Build history of the part. All positions in model axes, mm. Face numbers are marked on the shaded views. Give positions to 0.01 mm unless a question says otherwise; leave off trailing zeros. Loops run counter-clockwise (first coordinate to the right, second up) from the corner with the lowest first, then second, coordinate; pieces in that order, holes last. Notation, with made-up numbers: M 72.25,17 L 98.25,17 A21 cw 98.25,41 Z; hole C 71.5,77.25 d9. An arc over 180 degrees is marked long. Put each result on its own line as item: value.
```python
from build123d import *

# Parameters (mm, degrees)
SKETCH1_R           = 2.5
BOSS_EXTRUDE1_DEPTH = 30
FILLET1_R           = 5


with BuildPart() as part:
    # Sketch1 → Boss-Extrude1 (new body)
    with BuildSketch(Plane(origin=(0, 0, 0), x_dir=(1, 0, 0), z_dir=(0, 1, 0))):
        with BuildLine():
            Line((0, 5), (20, 5))
            Line((20, 5), (20, -5))
            Line((20, -5), (0, -5))
            ThreePointArc((0, -5), (-5, 0), (0, 5))
        make_face()
        with Locations(Location((0, 0, 0), (0, 0, 270))):
            Circle(SKETCH1_R, mode=Mode.SUBTRACT)
    extrude(amount=BOSS_EXTRUDE1_DEPTH)

    # Fillet1
    fillet1_edges = [part.edges().sort_by_distance(p)[0] for p in [
        (20, 15, 5),
    ]]
    fillet(fillet1_edges, radius=FILLET1_R)


solid = part.part
```
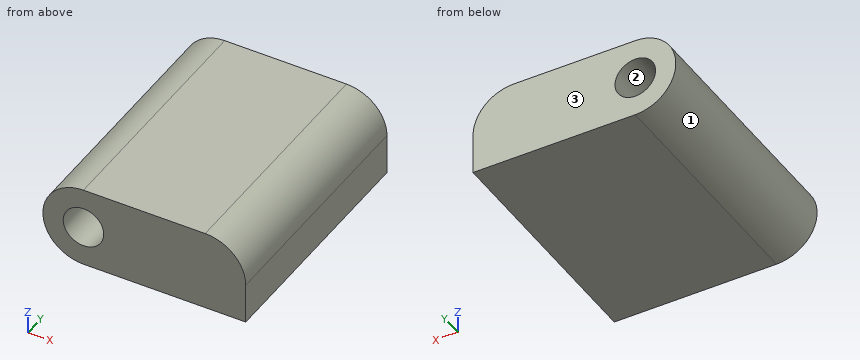
Q1. Slice it at C-C (z = -1.5). List the corners of the cut face in (x, y).
Here are the results:
outline: M -4.77,0 L -2,0 L -2,30 L -4.77,30 Z; M 2,0 L 20,0 L 20,30 L 2,30 Z
Q2. Slice it at D-D (z = 3). List the corners of the cut face in (x, y), and give its area (3 significant figures).
Here are the results:
outline: M -4,0 L 19,0 L 19,30 L -4,30 Z
area: 690 mm²
Q3. Mould opens along Z. For the marked faces 1, 2 and 3 say: pulls with the +Z half, pulls with the -Z half, needs draft (parallel to the pull), parting line crosses it, or undercut.
Here are the results:
face 1: parting line crosses it
face 2: undercut
face 3: needs draft
Q4. Slice it at B-B (y = 25.75). List the corners of the cut face in (x, z).
Here are the results:
outline: M 0,-5 L 20,-5 L 20,0 A5 ccw 15,5 L 0,5 A5 ccw Z; hole C 0,0 d5
Q5. Slice it at A-A (x = 1.75). List the corners of the cut face in (y, z).
Here are the results:
outline: M 0,-5 L 30,-5 L 30,-1.79 L 0,-1.79 Z; M 0,1.79 L 30,1.79 L 30,5 L 0,5 Z
Q6. Probe line 1 (Z direction, x = 0.75, y = 13); line 2 (X direction, y = 16, z = 0.25); line 3 (X direction, y = 22.75, z = 2.25). List the from-to ranges inside material, lowest first. Write a range as from..to.
Here are the results:
line 1: -5..-2.38, 2.38..5
line 2: -4.99..-2.49, 2.49..19.99
line 3: -4.47..-1.09, 1.09..19.47
